Work out the finished part from the listing and answer in its coordinate system (mm). A direction names the side the tool comes from. Round coordinates to 2 decimals unless told otherwise and drop trailing zeros. Order: outer loops, then holes, each group sorted by start corner. A loop starts at its lowest first (then second) coordinate and runs counter-clockwise, first axis right, second up. Notation, with made-up numbers: (67, 77) -> (86, 77) arc R25 cw to (86, 99) -> close; hole circle Ø9 at (78.5, -5.75). An arc over 180 degrees is marked (long way). Use one line per item in the form item = value.
```python
from build123d import *

# Parameters (mm, degrees)
F0_W     = 7.8999367909
F0_H     = 15
F0_W_2   = 1.9381828606
F0_H_2   = 9
F1_DEPTH = 2
F2_R     = 5.08
F3_D     = 1.2
F3_DEPTH = 12.7
F3_TIP   = 0.3605163714


with BuildPart() as f1:
    # F0 (on Front) → F1 (new body)
    with BuildSketch(Plane.XZ):
        with Locations((18.8592814558, -0.3737040295)):
            Rectangle(F0_W, F0_H)
        Polygon((-12.1191004291, -7.8737040295), (14.9093130603, -7.8737040295), (14.9093130603, 7.1262959705), (-12.1191004291, 7.1262959705), (-12.1191004291, -1.8737040295), align=None)
        with Locations((-13.0881918594, 2.6262959705)):
            Rectangle(F0_W_2, F0_H_2)
    extrude(amount=F1_DEPTH)

    # F2
    f2_edges = [f1.edges().sort_by_distance(p)[0] for p in [
        (22.80925, -1, -7.873704),
        (22.80925, -1, 7.126296),
    ]]
    fillet(f2_edges, radius=F2_R)

    # F3
    with Locations(Plane(origin=(0, 0, 0), x_dir=(1, 0, 0), z_dir=(0, 1, 0))):
        with Locations((19.0357716603, 0.2653072295)):
            Hole(F3_D / 2, depth=F3_DEPTH)
            with Locations((0, 0, -(F3_DEPTH + F3_TIP / 2))):  # 118° drill point
                Cone(0, F3_D / 2, F3_TIP, mode=Mode.SUBTRACT)


solid = f1.part
```
Item 1: Determine the mould class of faces 3 (the cylindrical face through (18.48, -1.01, -0.04)), 4 (the flat face through (2, -1, 7.126)), 5 (the cylindrical face through (21.361, -1.014, -6.346)), 6 (the flat face through (-12.119, -1, -5)) for opening direction X: released by +X, released by -X, zero draft, split by the parting line, or undercut.
Findings:
face_3 = undercut
face_4 = zero draft
face_5 = released by +X
face_6 = released by -X
Item 2: Consider line 1 along Z through (x, y) = (19, -0.95); line 2 along X through (y, z) = (-1.4, -3); line 3 along X through (y, z) = (-1.15, -5.25). Determine where each line is inside the solid, lowest interval first.
Findings:
line_1 = -7.71 to -0.86, 0.33 to 6.96
line_2 = -12.12 to 22.81
line_3 = -12.12 to 22.18
Item 3: For faces 1 (the flat face through (-14.057, -1, 3)), 2 (the flat face through (-13, -1, -1.874)), determine the directions among +Z, -Z, +X, -X, +Y, -Y from which every point of the face is accessible in a straight line to the end or side of a thin tool.
Findings:
face_1 = +Z, -Z, -X, +Y, -Y
face_2 = -Z, -X, +Y, -Y
Item 4: Flat-ended cylindrical pins translate along their axes: P1, Ø0.7, axis at x = 19.04, z = -0.27, coming from the -Y side; P2, Ø1, axis at x = -13, y = -1, coming from the -Z side. Find the tip coordinate at first contact, or state that the pin passes through.
Findings:
P1 = through
P2 = -1.87
Item 5: The part is cut by section C-C, the plane z = 6.25. Give the vertices of the cut face in (x, y), and give its area (3 significant figures).
Findings:
outline = (-14.06, -2) -> (20.58, -2) -> (20.58, 0) -> (-14.06, 0) -> close
area = 69.3 mm^2
Item 6: The part is cut by section A-A, the plane y = -0.45. Give the vertices of the cut face in (x, z).
Findings:
outline = (-14.06, -1.87) -> (-12.12, -1.87) -> (-12.12, -7.87) -> (17.73, -7.87) arc R5.08 ccw to (22.81, -2.79) -> (22.81, 2.05) arc R5.08 ccw to (17.73, 7.13) -> (-14.06, 7.13) -> close; hole circle Ø1.2 at (19.04, -0.27)
Item 7: The part is cut by section B-B, the plane z = -3.5. Give the vertices of the cut face in (x, y), and give its area (3 significant figures).
Findings:
outline = (-12.12, -2) -> (22.76, -2) -> (22.76, 0) -> (-12.12, 0) -> close
area = 69.8 mm^2
